Geometry: see drawing. Coordinates: mm, zero at the bounding-box minimum. A direction names the side the tool comes from. Give positions to 0.01 mm unless a question says otherwise; leave off trailing zeros. Order: outer loops, then holes, each group sorted by start corner. A loop starts at its lowest first (then second) coordinate and runs counter-clockwise, first axis right, second up. Notation, with made-up numbers: (12.25, -2) - (23.25, -2) arc R21 ccw to (23.25, 8) - close; hole circle Ø2 at (-27.75, 44). An arc over 180 degrees is marked (long way). One line per item, written item: value.
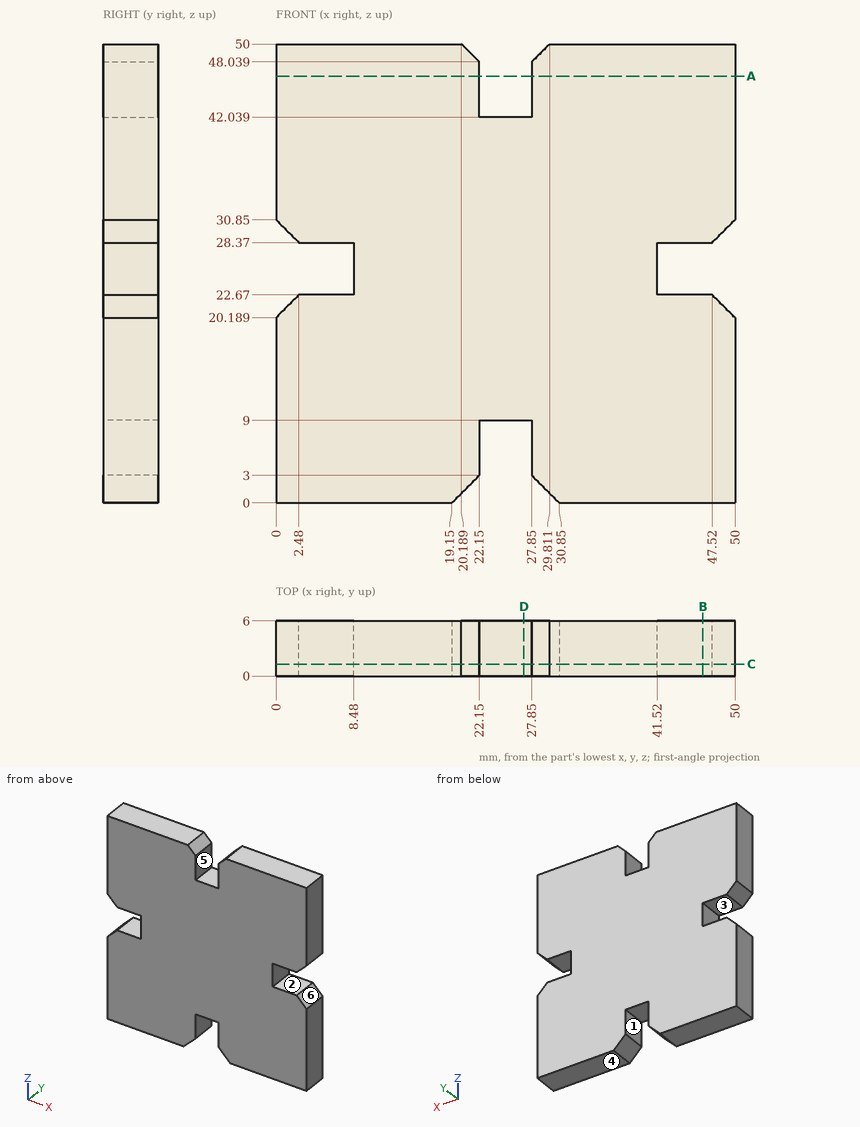
1) Section A-A, the plane z = 46.5. Return loops of the section in (x, y).
Answers below:
outline: (0, 0) - (22.15, 0) - (22.15, 6) - (0, 6) - close; (27.85, 0) - (50, 0) - (50, 6) - (27.85, 6) - close
2) Section D-D, the plane x = 27. Return loops of the section in (y, z), then the cut area to 3 significant figures.
Answers below:
outline: (0, 9) - (6, 9) - (6, 42.04) - (0, 42.04) - close
area: 198 mm^2
3) Material intervals for line 1 along X through (y, z) = (3.8, 5.5); line 2 along Z through (x, y) = (4, 1.65), sorted ascending.
Answers below:
line 1: 0 to 22.15, 27.85 to 50
line 2: 0 to 22.67, 28.37 to 50
4) Mould query, pull axis Z, two halves, no side actions, for the marked faces 4, 5 and 6. Classes: released by +Z, released by -Z, zero draft, split by the parting line, or undercut.
Answers below:
face 4: released by -Z
face 5: zero draft
face 6: undercut
5) Set-up query: the marked faces 1, 2 and 3. Return all of +Z, -Z, +X, -X, +Y, -Y with unobstructed straight access to the full face (end or side cutting, diameter ignored); none if empty.
Answers below:
face 1: -Z, +Y, -Y
face 2: +X, +Y, -Y
face 3: -X, +Y, -Y
6) Section C-C, the plane y = 1.3. Return loops of the section in (x, z).
Answers below:
outline: (0, 0) - (19.15, 0) - (22.15, 3) - (22.15, 9) - (27.85, 9) - (27.85, 3) - (30.85, 0) - (50, 0) - (50, 20.19) - (47.52, 22.67) - (41.52, 22.67) - (41.52, 28.37) - (47.52, 28.37) - (50, 30.85) - (50, 50) - (29.81, 50) - (27.85, 48.04) - (27.85, 42.04) - (22.15, 42.04) - (22.15, 48.04) - (20.19, 50) - (0, 50) - (0, 30.85) - (2.48, 28.37) - (8.48, 28.37) - (8.48, 22.67) - (2.48, 22.67) - (0, 20.19) - close
7) Section B-B, the plane x = 46.5. Return loops of the section in (y, z), then the cut area to 3 significant figures.
Answers below:
outline: (0, 0) - (6, 0) - (6, 22.67) - (0, 22.67) - close; (0, 28.37) - (6, 28.37) - (6, 50) - (0, 50) - close
area: 266 mm^2
8) First-contact query: pin 1 (3 mm diameter, centred on x = 26, y = 4, fed in from -Z). Flat tip, straight axial feed; report the tip coordinate or a pass-through.
Answers below:
pin 1: z = 9
